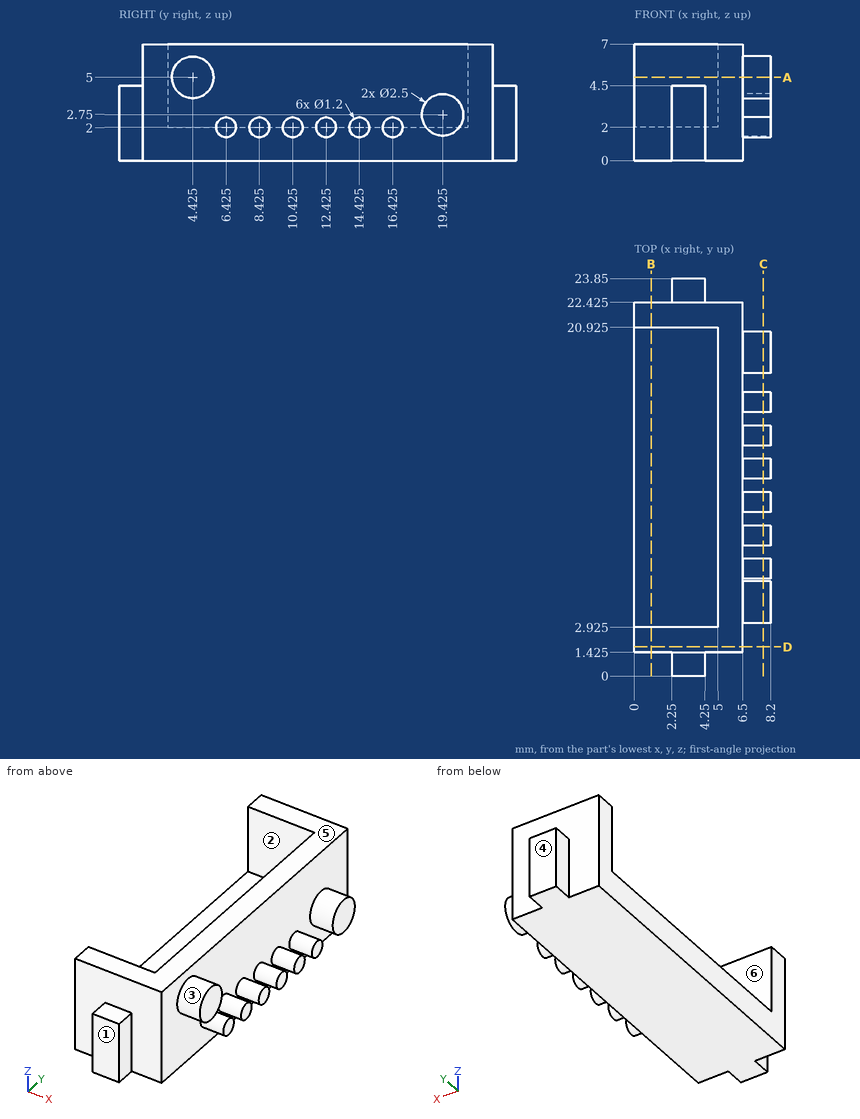
Input: dimensioned drawing with shaded views. Units: mm. Origin: part minimum x, y, z. A direction names the side the tool comes from. Give positions to 0.01 mm unless a question says otherwise; leave off trailing zeros. Order: outer loops, then holes, each group sorted by start corner. A loop starts at its lowest first (then second) coordinate and runs counter-clockwise, first axis right, second up. Notation, with made-up numbers: (-11.75, -8.5) -> (47.25, -8.5) arc R28 ccw to (47.25, 10.5) -> close; hole circle Ø1 at (-29.75, -20.5). An arc over 180 degrees is marked (long way). Answer as a JSON object with one key per item and string values.
Q1. First-contact query: pin 1 (2 mm diameter, centred on x = 6, z = 3.5, fed in from +Y) (3 decimals); pin 2 (0.7 mm diameter, centred on y = 0.5, z = 2.5, fed in from +X); pin 3 (1.1 mm diameter, centred on y = 0.5, z = 2, fed in from -X). Flat tips, straight axial feed; report the tip coordinate or a pass-through.
Entries:
{"pin 1": "stops at y = 22.425", "pin 2": "stops at x = 4.25", "pin 3": "stops at x = 2.25"}
Q2. Section B-B (x = 1). Output: boundary loops of the cut face in (y, z) (3 decimals).
Entries:
{"outline": "(1.425, 0) -> (22.425, 0) -> (22.425, 7) -> (20.925, 7) -> (20.925, 2) -> (2.925, 2) -> (2.925, 7) -> (1.425, 7) -> close"}
Q3. Section D-D (y = 1.75). Output: boundary loops of the cut face in (x, z), plus the area to 3 significant figures.
Entries:
{"outline": "(0, 0) -> (6.5, 0) -> (6.5, 7) -> (0, 7) -> close", "area": "45.5 mm^2"}
Q4. Material intervals for probe 1 along Y at (x, z) = (3.5, 6.75) (3 decimals); probe 2 along X at (y, z) = (20.5, 2.75); probe 3 along Y at (x, z) = (3.5, 2.5) (3 decimals), sorted ascending.
Entries:
{"probe 1": "y = 1.425 to 2.925, 20.925 to 22.425", "probe 2": "x = 5 to 8.2", "probe 3": "y = 0 to 2.925, 20.925 to 23.85"}
Q5. Access query for the marked faces 1, 2 and 3. Directions: +Z, -Z, +X, -X, +Y, -Y. A direction counts if a zero-diameter tool reaches every point of the face in a straight line with its end or side. Return the directions, or none.
Entries:
{"face 1": "+Z, -Z, +X, -X, -Y", "face 2": "+Z, -X", "face 3": "+X"}
Q6. Section C-C (x = 7.75). Output: boundary loops of the cut face in (y, z) (3 decimals).
Entries:
{"outline": "circle Ø2.5 at (4.425, 5); circle Ø1.2 at (6.425, 2); circle Ø1.2 at (8.425, 2); circle Ø1.2 at (10.425, 2); circle Ø1.2 at (12.425, 2); circle Ø1.2 at (14.425, 2); circle Ø1.2 at (16.425, 2); circle Ø2.5 at (19.425, 2.75)"}
Q7. Draft query along Y for the marked faces 4, 5 and 6. Return one class per face: released by +Y, released by -Y, zero draft, split by the parting line, or undercut.
Entries:
{"face 4": "released by +Y", "face 5": "zero draft", "face 6": "undercut"}
Q8. Section A-A (z = 5). Output: boundary loops of the cut face in (x, y) (3 decimals), plus the area to 4 significant figures.
Entries:
{"outline": "(0, 1.425) -> (6.5, 1.425) -> (6.5, 3.175) -> (8.2, 3.175) -> (8.2, 5.675) -> (6.5, 5.675) -> (6.5, 22.425) -> (0, 22.425) -> (0, 20.925) -> (5, 20.925) -> (5, 2.925) -> (0, 2.925) -> close", "area": "50.75 mm^2"}
